```python
from build123d import *

# Parameters (mm, degrees)
SKETCH_1_R             = 4
EXTRUDE_1_DEPTH        = 4
CUT_EXTRUDE_START      = -10
CUT_EXTRUDE_1_DEPTH    = 10
CUT_EXTRUDE_2_DEPTH    = 1
FILLET_1_R             = 1
SKETCH_5_R             = 7.5
SKETCH_5_R_2           = 4
EXTRUDE_2_DEPTH        = 0.25
FILLET_1_OF_MIRROR_1_R = 1
SKETCH_4_R             = 7
SKETCH_4_R_2           = 5
CUT_EXTRUDE_3_DEPTH    = 1
FILLET_2_R             = 1
CUT_EXTRUDE_START_2    = -0.25
SKETCH_6_R             = 7.5
CUT_EXTRUDE_4_DEPTH    = 0.25


with BuildPart() as part:
    # 草图1 → 凸台-拉伸1 (new body)
    with BuildSketch(Plane.XY):
        with BuildLine():
            Line((-30, 8), (30, 8))
            ThreePointArc((30, 8), (38, 0), (30, -8))
            Line((30, -8), (-30, -8))
            ThreePointArc((-30, -8), (-38, 0), (-30, 8))
        make_face()
        with Locations((-30, 0)):
            Circle(SKETCH_1_R, mode=Mode.SUBTRACT)
        with Locations((30, 0)):
            Circle(SKETCH_1_R, mode=Mode.SUBTRACT)
    extrude(amount=EXTRUDE_1_DEPTH)

    # 草图2 → 切除-拉伸1 (cut)
    with BuildSketch(Plane.XY.offset(4).offset(CUT_EXTRUDE_START)):
        with BuildLine():
            Line((30, 8), (-30, 8))
            ThreePointArc((-30, 8), (-28.285581944, 7.814139155), (-26.650824686, 7.265192683))
            ThreePointArc((-26.650824686, 7.265192683), (-20.520484967, 5.206643412), (-14.091417259, 4.509665243))
            Line((-14.091417259, 4.509665243), (14.091417259, 4.509665243))
            ThreePointArc((14.091417259, 4.509665243), (20.520484967, 5.206643412), (26.650824686, 7.265192683))
            ThreePointArc((26.650824686, 7.265192683), (28.285581944, 7.814139155), (30, 8))
        make_face()
        with BuildLine():
            Line((14.091417259, -4.509665243), (-14.091417259, -4.509665243))
            ThreePointArc((-14.091417259, -4.509665243), (-20.520484967, -5.206643412), (-26.650824686, -7.265192683))
            ThreePointArc((-26.650824686, -7.265192683), (-28.285581944, -7.814139155), (-30, -8))
            Line((-30, -8), (30, -8))
            ThreePointArc((30, -8), (28.285581944, -7.814139155), (26.650824686, -7.265192683))
            ThreePointArc((26.650824686, -7.265192683), (20.520484967, -5.206643412), (14.091417259, -4.509665243))
        make_face()
    extrude(amount=CUT_EXTRUDE_1_DEPTH, mode=Mode.SUBTRACT)

    # 草图3 → 切除-拉伸2 (cut)
    with BuildSketch(Plane.XY.offset(4)):
        with BuildLine():
            ThreePointArc((-23.634199351, -3.965675491), (-18.918027247, -2.875761974), (-14.091417259, -2.509665243))
            Line((-14.091417259, -2.509665243), (14.091417259, -2.509665243))
            ThreePointArc((14.091417259, -2.509665243), (18.918027247, -2.875761974), (23.634199351, -3.965675491))
            ThreePointArc((23.634199351, -3.965675491), (22.5, 0), (23.634199351, 3.965675491))
            ThreePointArc((23.634199351, 3.965675491), (18.918027247, 2.875761974), (14.091417259, 2.509665243))
            Line((14.091417259, 2.509665243), (-14.091417259, 2.509665243))
            ThreePointArc((-14.091417259, 2.509665243), (-18.918027247, 2.875761974), (-23.634199351, 3.965675491))
            ThreePointArc((-23.634199351, 3.965675491), (-22.789122631, 2.062340313), (-22.5, 0))
            ThreePointArc((-22.5, 0), (-22.789122631, -2.062340313), (-23.634199351, -3.965675491))
        make_face()
    cut_extrude_2 = extrude(amount=-CUT_EXTRUDE_2_DEPTH, mode=Mode.SUBTRACT)

    # 圆角1
    fillet_1_edges = [part.edges().sort_by_distance(p)[0] for p in [
        (23.634199351, -3.965675491, 3.5),
        (-23.634199351, -3.965675491, 3.5),
        (-23.634199351, 3.965675491, 3.5),
        (23.634199351, 3.965675491, 3.5),
    ]]
    fillet(fillet_1_edges, radius=FILLET_1_R)

    # 草图5 → 凸台-拉伸2 (add)
    # profile 1 of 2: a face of its own
    with BuildSketch(Plane(origin=(0, 0, 0), x_dir=(-1, 0, 0), z_dir=(0, 0, -1))):
        with Locations((30, 0)):
            Circle(SKETCH_5_R)
        with Locations((30, 0)):
            Circle(SKETCH_5_R_2, mode=Mode.SUBTRACT)
    # profile 2 of 2: a face of its own
    with BuildSketch(Plane(origin=(0, 0, 0), x_dir=(-1, 0, 0), z_dir=(0, 0, -1))):
        with Locations(Location((-30, 0, 0), (0, 0, 180))):
            Circle(SKETCH_5_R)
        with Locations((-30, 0)):
            Circle(SKETCH_5_R_2, mode=Mode.SUBTRACT)
    extrude(amount=EXTRUDE_2_DEPTH)

    # 镜向1: 切除-拉伸2 across plane
    add(cut_extrude_2.mirror(Plane(origin=(0, 0, 2), x_dir=(1, 0, 0), z_dir=(0, 0, -1))), mode=Mode.SUBTRACT)

    # 圆角1 of 镜向1
    fillet_1_of_mirror_1_edges = [part.edges().sort_by_distance(p)[0] for p in [
        (23.634199351, -3.965675491, 0.5),
        (-23.634199351, -3.965675491, 0.5),
        (-23.634199351, 3.965675491, 0.5),
        (23.634199351, 3.965675491, 0.5),
    ]]
    fillet(fillet_1_of_mirror_1_edges, radius=FILLET_1_OF_MIRROR_1_R)

    # 草图4 → 切除-拉伸3 (cut)
    # profile 1 of 2: a face of its own
    with BuildSketch(Plane.XY.offset(-0.25)):
        with Locations((30, 0)):
            Circle(SKETCH_4_R)
        with Locations((30, 0)):
            Circle(SKETCH_4_R_2, mode=Mode.SUBTRACT)
    # profile 2 of 2: a face of its own
    with BuildSketch(Plane.XY.offset(-0.25)):
        with Locations((-30, 0)):
            Circle(SKETCH_4_R)
        with Locations((-30, 0)):
            Circle(SKETCH_4_R_2, mode=Mode.SUBTRACT)
    extrude(amount=CUT_EXTRUDE_3_DEPTH, mode=Mode.SUBTRACT)

    # 圆角2
    fillet_2_edges = [part.edges().sort_by_distance(p)[0] for p in [
        (23, 0, 0.75),
        (25, 0, 0.75),
        (-37, 0, 0.75),
        (-35, 0, 0.75),
    ]]
    fillet(fillet_2_edges, radius=FILLET_2_R - 0.0001)  # a hair under: the kernel refuses the full size

    # 草图6 → 切除-拉伸4 (cut)
    with BuildSketch(Plane(origin=(0, 0, -0.25), x_dir=(-1, 0, 0), z_dir=(0, 0, -1)).offset(CUT_EXTRUDE_START_2)):
        with Locations((30, 0)):
            Circle(SKETCH_6_R)
        with Locations((-30, 0)):
            Circle(SKETCH_6_R)
    extrude(amount=CUT_EXTRUDE_4_DEPTH, mode=Mode.SUBTRACT)


solid = part.part
```
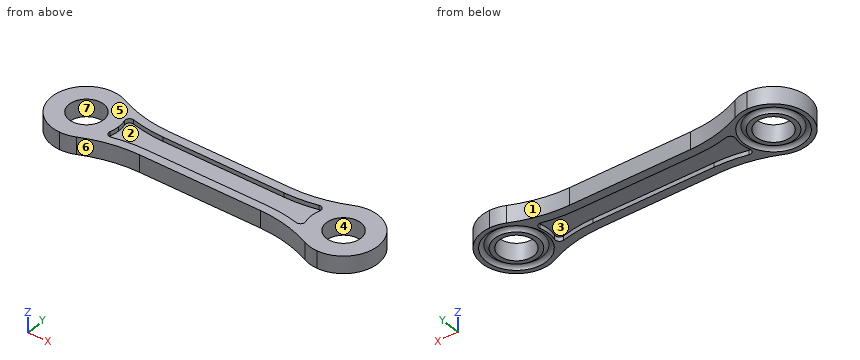
Can you work these out from the model? Positions are in its coordinate system, mm. Face numbers are marked on the shaded views. A direction names the side the tool comes from. Round coordinates to 2 decimals unless told otherwise and drop trailing zeros. Order: outer loops, then holes, each group sorted by start corner. A loop starts at its lowest first (then second) coordinate and runs counter-clockwise, first axis right, second up. Notation, with made-up numbers: (65, 21.5) -> (110, 21.5) arc R19 cw to (110, 36.5) -> close; hole circle Ø5 at (-33.5, 66). An arc over 180 degrees is marked (long way). Return JSON: item names as keys, results as strings. Group by question number.
1. Which directions (+Z, -Z, +X, -X, +Y, -Y) give clear straight access to the entire face, cutting with the end or side of a thin tool? Please do the marked faces 1, 2, 3 and 4.
2. If we section it at A-A, the plane z = 1.85: Write out the boundary of the cut face in (x, y), then the cut area to 3 significant figures.
3. If we section it at C-C, the plane x = 17.5: Write out the boundary of the cut face in (y, z).
4. We'd pull the mould along Y, two halves only. Please class the marked faces 5, 6 and 7: released by +Y, released by -Y, zero draft, split by the parting line, or undercut.
5. If we section it at B-B, the plane x = -9: Write out the boundary of the cut face in (y, z), then the cut area to 3 significant figures.
6. I need wall thicknesses on line 1 (Y direction, x = -30, z = 1.3); line 2 (X direction, y = -2.5, z = 2.95); line 3 (Y direction, x = 14, z = 0.9). Which ranges of each line are inside material? Lowest first, please. Write a range as [from, to].
7. Will these pins go through, and if not, where does the flat tip stop? pin 1 (3.5 mm diameter, centred on x = -8.5, y = -1.5, fed in from -Z); pin 2 (1.1 mm diameter, centred on x = 7, z = 3.5, fed in from -Y); pin 3 (1 mm diameter, centred on x = 18, z = 1.5, fed in from +Y); pin 4 (0.5 mm diameter, centred on x = -7, z = 0.5, fed in from +Y).
Output values:
{
 "1": {"face 1": "+Z, -Z, +Y", "face 2": "+Z", "face 3": "-Z", "face 4": "+Z, -Z"},
 "2": {"outline": "(-26.65, -7.27) arc R30 cw to (-14.09, -4.51) -> (14.09, -4.51) arc R30 cw to (26.65, -7.27) arc R8 ccw (long way) to (26.65, 7.27) arc R30 cw to (14.09, 4.51) -> (-14.09, 4.51) arc R30 cw to (-26.65, 7.27) arc R8 ccw (long way) to start; hole circle Ø8 at (-30, 0); hole circle Ø8 at (30, 0)", "area": "730 mm²"},
 "3": {"outline": "(-4.7, 0) -> (-2.69, 0) -> (-2.69, 1) -> (2.69, 1) -> (2.69, 0) -> (4.7, 0) -> (4.7, 4) -> (2.69, 4) -> (2.69, 3) -> (-2.69, 3) -> (-2.69, 4) -> (-4.7, 4) -> close"},
 "4": {"face 5": "zero draft", "face 6": "released by -Y", "face 7": "undercut"},
 "5": {"outline": "(-4.51, 0) -> (-2.51, 0) -> (-2.51, 1) -> (2.51, 1) -> (2.51, 0) -> (4.51, 0) -> (4.51, 4) -> (2.51, 4) -> (2.51, 3) -> (-2.51, 3) -> (-2.51, 4) -> (-4.51, 4) -> close", "area": "26.0 mm²"},
 "6": {"line 1": "[-8, -4], [4, 8]", "line 2": "[-37.6, -33.12], [-26.88, 26.88], [33.12, 37.6]", "line 3": "[-4.51, -2.51], [2.51, 4.51]"},
 "7": {"pin 1": "z = 0", "pin 2": "y = -4.51", "pin 3": "y = 4.84", "pin 4": "y = 4.51"}
}
